Read the model definition and answer for the solid it produces. Units are mm, in the model's axes. Face numbers are marked on the shaded views. A direction names the side the tool comes from. Give positions to 0.01 mm unless a question says otherwise; leave off trailing zeros. Order: outer loops, then holes, each group sorted by start corner. A loop starts at its lowest first (then second) coordinate and runs counter-clockwise, first axis right, second up. Notation, with made-up numbers: (58, 23) - (104, 23) arc R32 ccw to (104, 56) - close; hole circle Ø4 at (-17.75, 66). An arc over 180 degrees is marked (long way). Write item = value, one per line.
Autodesk Inventor part; units mm, degrees
ref_plane "YZ Plane" through (0, 0, 0) normal (1, 0, 0) x (0, 1, 0)
ref_plane "XZ Plane" through (0, 0, 0) normal (0, 1, 0) x (-1, 0, 0)
ref_plane "XY Plane" through (0, 0, 0) normal (0, 0, 1) x (1, 0, 0)
sketch "Эскиз1" plane through (0, 0, 0) normal (0, 1, 0) x (-1, 0, 0)
  circle A0 centre (0, 0) radius 1.6
  circle A1 centre (0, -0.0001) radius 5
  line L0 (-40, -6.3417) -> (-40, 6.3417)
  line L1 (-40, 16) -> (-46.0917, 16)
  line L2 (-46.0917, -16) -> (-40, -16)
  line L3 (-40, -16) -> (-40, -9.6583)
  line L4 (-40, -6.3417) -> (-40, -9.6583)
  line L5 (-40, 9.6583) -> (-40, 6.3417)
  line L6 (-40, 9.6583) -> (-40, 16)
  line L7 (-40, 16) -> (-46.0917, 16)
  line L8 (-46.0917, 16) -> (-46.0917, -16)
  line L9 (-46.0917, -16) -> (-40, -16)
  line L10 (-40, -16) -> (-40, 16)
  circle A2 centre (0, -0.0001) radius 10
  arc A3 (-40, 16) -> (-0.0411, 9.9998) centre (-0.586, 142.4269) ccw
  arc A4 (-0.0411, -10) -> (-40, -16) centre (-0.5865, -142.4271) ccw
  point P0 (0, 0)
  dimension "d0" = 20
  dimension "d1" = 132.4282
  dimension "d2" = 132.4282
extrude "Выдавливание1" add sketch "Эскиз1" along normal blind 5 contours A1 | L4 L3 L2 L8 L1 L6 L5 L0 | L0 L5 L6 A3 A2 A4 L3 L4 | A2
sketch "Эскиз2" plane through (0, 0, 0) normal (0, -1, 0) x (1, 0, 0)
  circle A0 centre (42.5, -8) radius 1.25
  circle A1 centre (0, 0) radius 1.6
  line L0 (46.0917, -16) -> (40, -16)
  line L1 (46.0917, 16) -> (46.0917, -16)
  line L2 (40, 16) -> (46.0917, 16)
  arc A2 (0.0411, 9.9998) -> (40, 16) centre (0.586, 142.4269) ccw
  arc A3 (0.0411, 9.9998) -> (0.0411, -10) centre (0, -0.0001) ccw
  arc A4 (40, -16) -> (0.0411, -10) centre (0.5865, -142.4271) ccw
  circle A5 centre (42.5, 8) radius 1.25
  point P0 (0, 0)
extrude "Выдавливание2" cut sketch "Эскиз2" against normal blind 5 contours A0 | A5
sketch "Эскиз3" plane through (0, 0, 0) normal (0, -1, 0) x (1, 0, 0)
  line L0 (46.0917, 16) -> (46.0917, -16)
  arc A0 (40, -16) -> (0.0411, -10) centre (0.5865, -142.4271) ccw
  line L1 (46.0917, 16) -> (40, 16)
  line L2 (40, 16) -> (40, -16)
  line L3 (40, -16) -> (46.0917, -16)
  line L4 (46.0917, -16) -> (46.0917, 16)
  circle A1 centre (42.5, 8) radius 1.25
  circle A2 centre (42.5, 8) radius 1.25
  circle A3 centre (42.5, -8) radius 1.25
  circle A4 centre (42.5, -8) radius 1.25
  point P0 (0, 0)
extrude "Выдавливание3" add sketch "Эскиз3" along normal blind 18.8
chamfer "Фаска1" distance 10 angle 45 1 edges at (40, 0, 0)
sketch "Эскиз4" plane through (0, 5, 0) normal (0, 1, 0) x (1, 0, 0)
  circle A0 centre (42.5, -8) radius 1.25
  circle A1 centre (42.5, -8) radius 3
  circle A2 centre (42.5, 8) radius 1.25
  circle A3 centre (42.5, 8) radius 3
  point P0 (0, 0)
  dimension "d12" = 6
  dimension "d13" = 6
extrude "Выдавливание4" cut sketch "Эскиз4" against normal blind 20
chamfer "Фаска2" distance 2 angle 45 1 edges at (46.0917, 5, 0)
chamfer "Фаска3" distance 1 angle 45 3 edges at (44.0917, 5, 0) (44.0917, 5, 13.2715) (44.0917, 5, -13.2715)
equation "\"d2\" = d1"
properties part number "000.403 - Верхний рычаг"
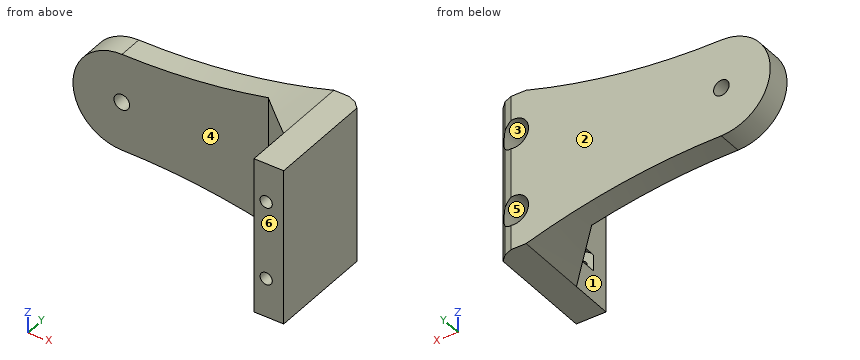
1. Section D-D (x = 3) is taken. Determine the outline of the cut face in (y, z), and give its area (3 significant figures).
Recorded:
outline = (0, -10.02) - (5, -10.02) - (5, 10.02) - (0, 10.02) - close
area = 100 mm^2
2. Section B-B (z = -8) is taken. Determine the outline of the cut face in (x, y), and give its area (3 significant figures).
Recorded:
outline = (-6, 0) - (30, 0) - (39.5, -9.5) - (39.5, 5) - (-6, 5) - close; (40, -18.8) - (41.25, -18.8) - (41.25, -15) - (40, -15) - close; (43.75, -18.8) - (46.09, -18.8) - (46.09, 3) - (45.5, 3.59) - (45.5, -15) - (43.75, -15) - close
area = 297 mm^2
3. Section A-A (z = 0) is taken. Determine the outline of the cut face in (x, y).
Recorded:
outline = (-10, 0) - (-1.6, 0) - (-1.6, 5) - (-10, 5) - close; (1.6, 0) - (30, 0) - (40, -10) - (40, -18.8) - (46.09, -18.8) - (46.09, 3) - (44.8, 4.29) - (43.09, 5) - (1.6, 5) - close
4. Determine the mould class of the marked faces 1, 2 and 3 for opening direction X: +X half, -X half, draft (parallel to the pull), parting line (faces both ways), or undercut.
Recorded:
face_1 = -X half
face_2 = draft
face_3 = undercut
5. Flat-ended cylindrical pins translate along their axes: pin 1 (6 mm diameter, centred on y = -2.5, z = 6.5, fed in from -X); pin 2 (6 mm diameter, centred on y = -15, z = 12.5, fed in from -X); pin 3 (4 mm diameter, centred on x = 19, z = 7, fed in from -Y); pin 4 (3.5 mm diameter, centred on x = 42.5, z = 8, fed in from -Y). Find the tip coordinate at first contact, or state that the pin passes through.
Recorded:
pin_1 = -8.75
pin_2 = 40
pin_3 = 0
pin_4 = -18.8
6. For the marked faces 4, 5 and 6, determine the directions among +Z, -Z, +X, -X, +Y, -Y from which every point of the face is accessible in a straight line to the end or side of a thin tool.
Recorded:
face_4 = +Z, -Z, -X, -Y
face_5 = +Y
face_6 = +Z, -Z, +X, -X, -Y
7. Straight lines are drawn through the part: L1, parallel to Z at x = 42.5, y = -5.5; L2, parallel to Z at x = 42.5, y = -16; L3, parallel to Z at x = 0, y = 2.05. For each, find the intervals that lie inside material, in ascending order. Write a range as [from, to].
Recorded:
L1 = [-16, -11], [-5, 5], [11, 16]
L2 = [-16, -9.25], [-6.75, 6.75], [9.25, 16]
L3 = [-10, -1.6], [1.6, 10]
8. Section C-C (y = -8.5) is taken. Determine the outline of the cut face in (x, z), and give its area (3 significant figures).
Recorded:
outline = (38.5, -15.54) arc R132.43 cw to (40, -16) - (46.09, -16) - (46.09, 16) - (40, 16) arc R132.43 cw to (38.5, 15.54) - close; hole circle Ø6 at (42.5, -8); hole circle Ø6 at (42.5, 8)
area = 186 mm^2
